Check sheet for the modelled part. Datum: model origin and axes. Units: mm. A direction names the side the tool comes from. Round coordinates to 2 decimals unless told otherwise and drop trailing zeros. Write each loop counter-clockwise with the first axis right and the second up, starting at its lowest first coordinate (ties: lowest second). Pieces come first, ordered by that corner, then holes. Notation, with made-up numbers: (19, -17) - (47, -17) arc R31 ccw to (47, 20) - close; hole circle Ø3 at (84, 18.25). An arc over 180 degrees is marked (long way). Use one line per item in the form item = value. Start each with the question number.
1) Gauge pin test, flat ends, axial feed: P1, Ø6, axis at x = 1.5, z = 6, coming from the +Y side; P2, Ø1.5, axis at x = 2, z = 5, coming from the -Y side; P3, Ø1.8, axis at x = -0.5, z = 30, coming from the -Y side. Record the tip position at first contact, or that the pin passes through.
2) Scan lines: probe 1 along Y at (x, z) = (1, 30.5); probe 2 along Z at (x, y) = (1.75, 3.5); probe 3 along Y at (x, z) = (-1.75, 11.5). Record each from-to range of solid material in increasing order.
3) Set-up check for faces 5 (the face through (-2, -1, 8.6)), 6 (the face through (0, -2.956, 29)), 7 (the face through (0, 2.956, 29)), 8 (the face through (0, -2.656, 29)), 9 (the face through (-0.69, -3.1, 11.71)): record each of +Z, -Z, +X, -X, +Y, -Y from which the full face is reachable in a straight line by a thin tool's end or side.
4) Draft check along Z on faces 1 (the face through (2.4, -2.4, 14.6)), 2 (the face through (-3.6, -2.8, 22.5)), 3 (the face through (0, -2, 6)), 4 (the face through (1, -2, 4)). Enter one of: +Z half, -Z half, draft (parallel to the pull), parting line (faces both ways), or undercut.
5) Section check A-A (z = 19). Record the boundary of the cut face in (x, y), then the cut area to 3 significant figures.
6) Section check B-B (z = 3). Record the boundary of the cut face in (x, y).
from build123d import *

# Parameters (mm, degrees)
F0_R      = 3
F1_DEPTH  = 4
F2_R      = 2
F3_DEPTH  = 4.6
F4_R      = 3.175
F5_DEPTH  = 6
F6_R      = 5.5
F7_DEPTH  = 4
F8_R      = 4.5612364212
F9_DEPTH  = 8
F11_R     = 1
F12_R     = 0.3
F13_W     = 3.5
F13_H     = 0.3
F14_DEPTH = 5.8
F15_R     = 1.5


# Not quite as in the source:
# - a fillet or chamfer that OpenCascade refuses, or shapes differently, is made with other operations: its cross-section is extruded or revolved along the edge and cut away or added


with BuildPart() as f1:
    # F0 (on Top) → F1 (new body)
    with BuildSketch(Plane.XY):
        Circle(F0_R)
    extrude(amount=F1_DEPTH)

    # F2 (on face) → F3 (join)
    with BuildSketch(Plane.XY.offset(4)):
        Circle(F2_R)
    extrude(amount=F3_DEPTH)

    # F4 (on face) → F5 (join)
    with BuildSketch(Plane.XY.offset(8.6)):
        Circle(F4_R)
    extrude(amount=F5_DEPTH)

    # F6 (on face) → F7 (join)
    with BuildSketch(Plane.XY.offset(14.6)):
        Circle(F6_R)
    extrude(amount=F7_DEPTH)

    # F8 (on face) → F9 (join)
    with BuildSketch(Plane.XY.offset(18.6)):
        Circle(F8_R)
    extrude(amount=F9_DEPTH)

    # F10: fillet of radius 3.2064860271 on 1 edges, made by hand

    # F10_s1 → F10_t2 (revolve, cut)
    with BuildSketch(Plane.XZ):
        with BuildLine():
            ThreePointArc((5.5, 16.3330664898), (5.256027516, 17.5598778645), (4.5612364212, 18.6))
            Line((4.5612364212, 18.6), (5.5, 18.6))
            Line((5.5, 18.6), (5.5, 16.3330664898))
        make_face()
    revolve(axis=Axis((0, 0, 18.6), (0, 0, 1)), mode=Mode.SUBTRACT)

    # F11
    f11_edges = [f1.edges().sort_by_distance(p)[0] for p in [
        (-3, 0, 0),
    ]]
    fillet(f11_edges, radius=F11_R)

    # F12
    f12_edges = [f1.edges().sort_by_distance(p)[0] for p in [
        (-3.175, 0, 8.6),
    ]]
    fillet(f12_edges, radius=F12_R)

    # F13 (on face) → F14 (join)
    with BuildSketch(Plane.XY.offset(26.6)):
        with Locations((0, 2.8059364047)):
            Rectangle(F13_W, F13_H)
        with Locations((0, -2.8059364047)):
            Rectangle(F13_W, F13_H)
    extrude(amount=F14_DEPTH)

    # F15
    f15_edges = [f1.edges().sort_by_distance(p)[0] for p in [
        (1.75, 2.805936, 32.4),
        (1.75, -2.805936, 32.4),
        (-1.75, -2.805936, 32.4),
        (-1.75, 2.805936, 32.4),
    ]]
    fillet(f15_edges, radius=F15_R)


solid = f1.part
Results are:
q1.P1 = 3.13
q1.P2 = -1.56
q1.P3 = -2.96
q2.probe_1 = -2.96 to -2.66, 2.66 to 2.96
q2.probe_2 = 14.6 to 26.6
q2.probe_3 = -2.65 to 2.65
q3.face_5 = none
q3.face_6 = +Z, +X, -X, -Y
q3.face_7 = +Z, +X, -X, +Y
q3.face_8 = +Z, +X, -X
q3.face_9 = -Z
q4.face_1 = -Z half
q4.face_2 = draft
q4.face_3 = undercut
q4.face_4 = undercut
q5.outline = circle Ø9.12 at (0, 0)
q5.area = 65.4 mm²
q6.outline = circle Ø6 at (0, 0)
